Verification items for the finished model (mm, model axes). Give positions to 0.01 mm unless a question says otherwise; leave off trailing zeros. Loops run counter-clockwise (first coordinate to the right, second up) from the corner with the lowest first, then second, coordinate; pieces in that order, holes last. Notation, with made-up numbers: (52, 33.25) - (70, 33.25) arc R24 cw to (70, 64.25) - close; hole circle Ø10 at (71, -35). An arc over 180 degrees is marked (long way). One line per item, written item: value. Start each with the question number.
1. Sectioned sample at C-C (z = -0.95). Record the cut outline in (x, y), plus the area to 3 significant figures.
2. Sectioned sample at A-A (y = -32). Record the cut outline in (x, z).
3. Sectioned sample at B-B (x = 0.5). Record the cut outline in (y, z), plus the area to 4 significant figures.
4. Scan lines: L1, parallel to Y at x = 35.5, z = -2.75; L2, parallel to X at y = -33.5, z = -2.1; L3, parallel to Y at x = 2.5, z = -1.25. Record each from-to range of solid material in increasing order. Write a range as [from, to].
from build123d import *

# Parameters (mm, degrees)
SKETCH_W              = 50
SKETCH_H              = 36
PAD_DEPTH             = 5.5
SKETCH001_R           = 2.25
HOLE_DEPTH            = 25
CHAMFER_SIZE          = 1
CLONE_PLACEMENT_ANGLE = 180


with BuildPart() as part:
    # Sketch → Pad (new body)
    with BuildSketch(Plane.XY):
        Rectangle(SKETCH_W, SKETCH_H)
    extrude(amount=-PAD_DEPTH)

    # Sketch001 → Hole (cut)
    with BuildSketch(Plane.XY):
        with Locations((-17.5, 12)):
            Circle(SKETCH001_R)
        with Locations((17.5, 12)):
            Circle(SKETCH001_R)
        with Locations((17.5, -12)):
            Circle(SKETCH001_R)
        with Locations((-17.5, -12)):
            Circle(SKETCH001_R)
    extrude(amount=-HOLE_DEPTH, mode=Mode.SUBTRACT)

    # Chamfer
    chamfer_edges = [part.edges().sort_by_distance(p)[0] for p in [
        (-25, -18, -2.75),
        (25, -18, -2.75),
        (-25, 18, -2.75),
        (25, 18, -2.75),
    ]]
    chamfer(chamfer_edges, length=CHAMFER_SIZE)


with BuildPart() as part_1:
    # Clone placement: moved
    add(part.part.moved(Location((18, -20, 0))).rotate(Axis((18, -20, 0), (0, 0, 1)), CLONE_PLACEMENT_ANGLE))


solid = part_1.part
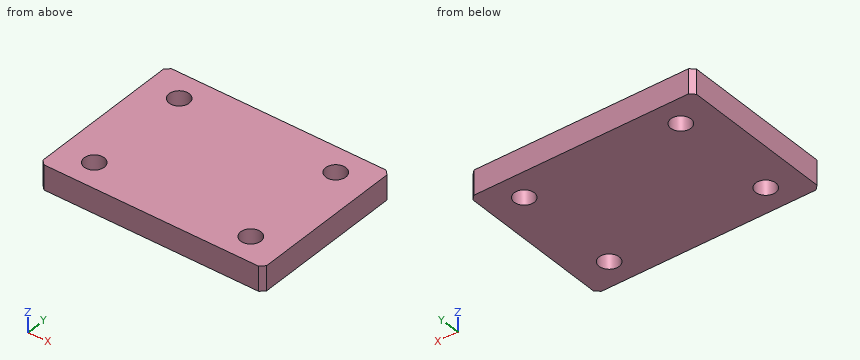
Results are:
1. outline: (-7, -37) - (-6, -38) - (42, -38) - (43, -37) - (43, -3) - (42, -2) - (-6, -2) - (-7, -3) - close; hole circle Ø4.5 at (0.5, -32); hole circle Ø4.5 at (0.5, -8); hole circle Ø4.5 at (35.5, -32); hole circle Ø4.5 at (35.5, -8)
1. area: 1,730 mm^2
2. outline: (-7, -5.5) - (-1.75, -5.5) - (-1.75, 0) - (-7, 0) - close; (2.75, -5.5) - (33.25, -5.5) - (33.25, 0) - (2.75, 0) - close; (37.75, -5.5) - (43, -5.5) - (43, 0) - (37.75, 0) - close
3. outline: (-38, -5.5) - (-34.25, -5.5) - (-34.25, 0) - (-38, 0) - close; (-29.75, -5.5) - (-10.25, -5.5) - (-10.25, 0) - (-29.75, 0) - close; (-5.75, -5.5) - (-2, -5.5) - (-2, 0) - (-5.75, 0) - close
3. area: 148.5 mm^2
4. L1: y = [-38, -34.25], [-29.75, -10.25], [-5.75, -2]
4. L2: x = [-7, -1.18], [2.18, 33.82], [37.18, 43]
4. L3: y = [-38, -33.03], [-30.97, -9.03], [-6.97, -2]
